The model under review builds one solid part; all positions refer to its coordinate system, in mm. A direction names the side the tool comes from. Give positions to 0.01 mm unless a question says otherwise; leave off trailing zeros. Order: outer loops, then holes, each group sorted by start corner. A loop starts at its lowest first (then second) coordinate and runs counter-clockwise, first axis right, second up. Notation, with made-up numbers: (86.25, 75.5) - (127.25, 75.5) arc R17 cw to (127.25, 96.5) - close; hole circle Ø8 at (42, 43). An arc over 180 degrees is marked (long way). Write item = value, one per line. Start each with the question number.
1. We need section D-D, the plane y = -18.6. Give the boundary of the cut face in (x, z), and give its area (3 significant figures).
2. Machinability: for faces 1 (the flat face through (46, -19, -6)), 2 (the flat face through (38, -20, -2)), which of the approach directions +Z, -Z, +X, -X, +Y, -Y give a long, thin tool a straight path to every point of the face, cutting with its end or side? Answer none if there is none.
3. We need section C-C, the plane z = -9. Give the boundary of the cut face in (x, y), and give its area (3 significant figures).
4. We need section A-A, the plane x = 46.5. Give the boundary of the cut face in (y, z), and give its area (4 significant figures).
5. We need section B-B, the plane y = -19.6. Give the boundary of the cut face in (x, z).
6. Mouldability with a two-part tool opening along Z and no side actions: class faces 3 (the cylindrical face through (46.15, -19.99, -10.56)), 4 (the cylindrical face through (39, -20, -10)), 5 (the flat face through (46, -16.5, 1)) as pulls with the +Z half, pulls with the -Z half, needs draft (parallel to the pull), parting line crosses it, or undercut.
7. For P1, Ø0.8, axis at x = 43, y = -17, coming from the -Z side; P2, Ø4, axis at x = 46.5, z = -9, coming from the +Y side, all flat-tipped, find the tip position at first contact; note any pin that passes through.
8. Wall thickness on probe 1 along Y at (x, z) = (52.75, -10.5); probe 2 along Z at (x, y) = (39, -18.95); probe 3 along Z at (x, y) = (46, -20.5): over which ranges is each line inside the solid? List them lowest first.
from build123d import *

# Parameters (mm, degrees)
CYLINDER074_R     = 1.6
CYLINDER074_DEPTH = 2
BOX188_W          = 17
BOX188_H          = 2
BOX188_DEPTH      = 14
FILLET042_R       = 5
BOX187_W          = 17
BOX187_H          = 2.5
BOX187_DEPTH      = 2.5


with BuildPart() as cylinder155:
    # Cylinder074 → Cylinder074 (new body)
    with BuildSketch(Plane(origin=(46.5, -19, -9), x_dir=(1, 0, 0), z_dir=(0, -1, 0))):
        Circle(CYLINDER074_R)
    extrude(amount=CYLINDER074_DEPTH)


with BuildPart() as fillet042:
    # Box188 → Box188 (new body)
    with BuildSketch(Plane(origin=(38, -21, -12), x_dir=(1, 0, 0), z_dir=(0, 0, 1))):
        with Locations((8.5, 1)):
            Rectangle(BOX188_W, BOX188_H)
    extrude(amount=BOX188_DEPTH)

    # Cut097: cut Cylinder155
    add(cylinder155.part, mode=Mode.SUBTRACT)

    # Fillet042
    fillet042_edges = [fillet042.edges().sort_by_distance(p)[0] for p in [
        (38, -20, -12),
        (55, -20, -12),
    ]]
    fillet(fillet042_edges, radius=FILLET042_R)


with BuildPart() as fusion059:
    # Box187 → Box187 (new body)
    with BuildSketch(Plane(origin=(38, -19, -0.5), x_dir=(1, 0, 0), z_dir=(0, 0, 1))):
        with Locations((8.5, 1.25)):
            Rectangle(BOX187_W, BOX187_H)
    extrude(amount=BOX187_DEPTH)

    # Fusion059: union Fillet042
    add(fillet042.part)


solid = fusion059.part
Model answer:
q1.outline = (38, -0.5) - (55, -0.5) - (55, 2) - (38, 2) - close
q1.area = 42.5 mm2
q2.face_1 = -Z, +X, -X, +Y
q2.face_2 = +Z, -Z, -X, +Y, -Y
q3.outline = (38.42, -21) - (44.9, -21) - (44.9, -19) - (38.42, -19) - close; (48.1, -21) - (54.58, -21) - (54.58, -19) - (48.1, -19) - close
q3.area = 25.9 mm2
q4.outline = (-21, -12) - (-19, -12) - (-19, -10.6) - (-21, -10.6) - close; (-21, -7.4) - (-19, -7.4) - (-19, -0.5) - (-16.5, -0.5) - (-16.5, 2) - (-21, 2) - close
q4.area = 27.85 mm2
q5.outline = (38, -7) arc R5 ccw to (43, -12) - (50, -12) arc R5 ccw to (55, -7) - (55, 2) - (38, 2) - close; hole circle Ø3.2 at (46.5, -9)
q6.face_3 = undercut
q6.face_4 = pulls with the -Z half
q6.face_5 = needs draft
q7.P1 = -0.5
q7.P2 = -19
q8.probe_1 = -21 to -19
q8.probe_2 = -0.5 to 2
q8.probe_3 = -12 to -10.52, -7.48 to 2
